from build123d import *

# Parameters (mm, degrees)
SKETCH_1_R          = 27.5
EXTRUDE_1_DEPTH     = 10
EXTRUDE_2_DEPTH     = 16
CUT_EXTRUDE_3_DEPTH = 20
FILLET_3_R          = 2
SKETCH_7_W          = 2
SKETCH_7_H          = 5
SKETCH_7_W_2        = 5
SKETCH_7_H_2        = 2
CUT_EXTRUDE_4_DEPTH = 20
SKETCH_8_R          = 1.75
CUT_EXTRUDE_5_DEPTH = 20
SKETCH_9_R          = 1.75
CUT_EXTRUDE_6_DEPTH = 30.5


with BuildPart() as part:
    # 草图1 → 凸台-拉伸1 (new body)
    with BuildSketch(Plane.XY):
        Circle(SKETCH_1_R)
    extrude(amount=EXTRUDE_1_DEPTH)

    # 草图2 → 凸台-拉伸2 (add)
    with BuildSketch(Plane.XY.offset(10)):
        with BuildLine():
            Line((-2.5, 5.5), (-2.5, 17.5))
            Line((-2.5, 17.5), (-2.5, 18.792973669))
            ThreePointArc((-2.5, 18.792973669), (-13.405705116, 13.405705116), (-18.792973669, 2.5))
            Line((-18.792973669, 2.5), (-17.5, 2.5))
            Line((-17.5, 2.5), (-5.5, 2.5))
            ThreePointArc((-5.5, 2.5), (-3.378679656, 3.378679656), (-2.5, 5.5))
        make_face()
        with BuildLine():
            Line((17.5, -2.5), (5.5, -2.5))
            ThreePointArc((5.5, -2.5), (3.378679656, -3.378679656), (2.5, -5.5))
            Line((2.5, -5.5), (2.5, -17.5))
            Line((2.5, -17.5), (2.5, -18.792973669))
            ThreePointArc((2.5, -18.792973669), (13.405705116, -13.405705116), (18.792973669, -2.5))
            Line((18.792973669, -2.5), (17.5, -2.5))
        make_face()
        with BuildLine():
            Line((17.5, 2.5), (5.5, 2.5))
            ThreePointArc((5.5, 2.5), (3.378679656, 3.378679656), (2.5, 5.5))
            Line((2.5, 5.5), (2.5, 17.5))
            Line((2.5, 17.5), (2.5, 18.792973669))
            ThreePointArc((2.5, 18.792973669), (13.405705116, 13.405705116), (18.792973669, 2.5))
            Line((18.792973669, 2.5), (17.5, 2.5))
        make_face()
        with BuildLine():
            Line((-2.5, -17.5), (-2.5, -5.5))
            ThreePointArc((-2.5, -5.5), (-3.378679656, -3.378679656), (-5.5, -2.5))
            Line((-5.5, -2.5), (-17.5, -2.5))
            Line((-17.5, -2.5), (-18.792973669, -2.5))
            ThreePointArc((-18.792973669, -2.5), (-13.405705116, -13.405705116), (-2.5, -18.792973669))
            Line((-2.5, -18.792973669), (-2.5, -17.5))
        make_face()
    extrude(amount=EXTRUDE_2_DEPTH)

    # 草图6 → 切除-拉伸3 (cut)
    with BuildSketch(Plane.XY.offset(10)):
        Polygon((18.792973669, -2.5), (5.5, -2.5), (2.5, -2.5), (2.5, -5.5), (2.5, -18.792973669), (-2.5, -18.792973669), (-2.5, -5.5), (-2.5, -2.5), (-5.5, -2.5), (-18.792973669, -2.5), (-18.792973669, 2.5), (-5.5, 2.5), (-2.5, 2.5), (-2.5, 5.5), (-2.5, 18.792973669), (2.5, 18.792973669), (2.5, 5.5), (2.5, 2.5), (5.5, 2.5), (18.792973669, 2.5), align=None)
    extrude(amount=-CUT_EXTRUDE_3_DEPTH, mode=Mode.SUBTRACT)

    # 圆角3
    # the kernel refuses this fillet: 2 mm, written as the material it adds along each edge
    with BuildSketch(Plane(origin=(0, 0, 10), x_dir=(-0.13117570134694587, -0.9913591354177037, 0), z_dir=(-0.9913591354177037, 0.13117570134694587, 0))) as fillet_3_piece_1_section:
        with BuildLine():
            CenterArc((18.958529988 + FILLET_3_R, FILLET_3_R), FILLET_3_R, 180, 90)
            Line((18.958529988, FILLET_3_R), (18.958529988, 0))
            Line((18.958529988, 0), (18.958529988 + FILLET_3_R, 0))
        make_face()
    fillet_3_piece_1 = revolve(axis=Axis((0, 0, 10), (0, 0, 1)), revolution_arc=105.075073745, mode=Mode.PRIVATE)
    fillet_3_piece_1 = split(fillet_3_piece_1, bisect_by=Plane(origin=(2.5, -19.248904349, 10.242638579), z_dir=(1, 0, 0)), keep=Keep.TOP, mode=Mode.PRIVATE)
    fillet_3_piece_1 = split(fillet_3_piece_1, bisect_by=Plane(origin=(4.206837789, -2.5, 10.242638579), z_dir=(0, -1, 0)), keep=Keep.TOP, mode=Mode.PRIVATE)
    add(fillet_3_piece_1)
    with BuildSketch(Plane(origin=(0, 0, 10), x_dir=(-0.13117570134694623, 0.9913591354177035, 0), z_dir=(-0.9913591354177035, -0.13117570134694623, 0))) as fillet_3_piece_2_section:
        with BuildLine():
            CenterArc((18.958529988 + FILLET_3_R, -FILLET_3_R), FILLET_3_R, 90, 90)
            Line((18.958529988, -FILLET_3_R), (18.958529988, 0))
            Line((18.958529988, 0), (18.958529988 + FILLET_3_R, 0))
        make_face()
    fillet_3_piece_2 = revolve(axis=Axis((0, 0, 10), (0, 0, -1)), revolution_arc=105.075073745, mode=Mode.PRIVATE)
    fillet_3_piece_2 = split(fillet_3_piece_2, bisect_by=Plane(origin=(4.206838505, 2.5, 10.242637951), z_dir=(0, 1, 0)), keep=Keep.TOP, mode=Mode.PRIVATE)
    fillet_3_piece_2 = split(fillet_3_piece_2, bisect_by=Plane(origin=(2.5, 19.24890412, 10.242637951), z_dir=(1, 0, 0)), keep=Keep.TOP, mode=Mode.PRIVATE)
    add(fillet_3_piece_2)
    with BuildSketch(Plane(origin=(0, 0, 10), x_dir=(-0.9913591354177035, 0.13117570134694678, 0), z_dir=(0.13117570134694678, 0.9913591354177035, 0))) as fillet_3_piece_3_section:
        with BuildLine():
            CenterArc((18.958529988 + FILLET_3_R, FILLET_3_R), FILLET_3_R, 180, 90)
            Line((18.958529988, FILLET_3_R), (18.958529988, 0))
            Line((18.958529988, 0), (18.958529988 + FILLET_3_R, 0))
        make_face()
    fillet_3_piece_3 = revolve(axis=Axis((0, 0, 10), (0, 0, 1)), revolution_arc=105.075073745, mode=Mode.PRIVATE)
    fillet_3_piece_3 = split(fillet_3_piece_3, bisect_by=Plane(origin=(-19.248904349, -2.5, 10.242638579), z_dir=(0, -1, 0)), keep=Keep.TOP, mode=Mode.PRIVATE)
    fillet_3_piece_3 = split(fillet_3_piece_3, bisect_by=Plane(origin=(-2.5, -4.206837789, 10.242638579), z_dir=(-1, 0, 0)), keep=Keep.TOP, mode=Mode.PRIVATE)
    add(fillet_3_piece_3)
    with BuildSketch(Plane(origin=(0, 0, 10), x_dir=(0.13117570134694595, 0.9913591354177037, 0), z_dir=(0.9913591354177037, -0.13117570134694595, 0))) as fillet_3_piece_4_section:
        with BuildLine():
            CenterArc((18.958529988 + FILLET_3_R, FILLET_3_R), FILLET_3_R, 180, 90)
            Line((18.958529988, FILLET_3_R), (18.958529988, 0))
            Line((18.958529988, 0), (18.958529988 + FILLET_3_R, 0))
        make_face()
    fillet_3_piece_4 = revolve(axis=Axis((0, 0, 10), (0, 0, 1)), revolution_arc=105.075073745, mode=Mode.PRIVATE)
    fillet_3_piece_4 = split(fillet_3_piece_4, bisect_by=Plane(origin=(-2.5, 19.248904349, 10.242638579), z_dir=(-1, 0, 0)), keep=Keep.TOP, mode=Mode.PRIVATE)
    fillet_3_piece_4 = split(fillet_3_piece_4, bisect_by=Plane(origin=(-4.206837789, 2.5, 10.242638579), z_dir=(0, 1, 0)), keep=Keep.TOP, mode=Mode.PRIVATE)
    add(fillet_3_piece_4)

    # 草图7 → 切除-拉伸4 (cut)
    with BuildSketch(Plane(origin=(0, 0, 0), x_dir=(-1, 0, 0), z_dir=(0, 0, -1))):
        with Locations((19.792973669, 0)):
            Rectangle(SKETCH_7_W, SKETCH_7_H)
        with Locations((0, -19.792973669)):
            Rectangle(SKETCH_7_W_2, SKETCH_7_H_2)
        with Locations((-19.792973669, 0)):
            Rectangle(SKETCH_7_W, SKETCH_7_H)
        with Locations((0, 19.792973669)):
            Rectangle(SKETCH_7_W_2, SKETCH_7_H_2)
    extrude(amount=-CUT_EXTRUDE_4_DEPTH, mode=Mode.SUBTRACT)

    # 草图8 → 切除-拉伸5 (cut)
    with BuildSketch(Plane.XY.offset(10)):
        with Locations((0, 24.460175936)):
            Circle(SKETCH_8_R)
        with Locations((24.460175936, 0)):
            Circle(SKETCH_8_R)
        with Locations((0, -24.460175936)):
            Circle(SKETCH_8_R)
        with Locations((-24.460175936, 0)):
            Circle(SKETCH_8_R)
    extrude(amount=-CUT_EXTRUDE_5_DEPTH, mode=Mode.SUBTRACT)

    # 草图9 → 切除-拉伸6 (cut, symmetric)
    with BuildSketch(Plane(origin=(0, 0, 0), x_dir=(1, 0, 0), z_dir=(0, 1, 0))):
        with Locations(Location((-10.646486834, -19, 0), (0, 0, 270))):
            Circle(SKETCH_9_R)
        with Locations(Location((10.646486834, -19, 0), (0, 0, 270))):
            Circle(SKETCH_9_R)
    extrude(amount=CUT_EXTRUDE_6_DEPTH, both=True, mode=Mode.SUBTRACT)


solid = part.part
Can you work these out from the model? Positions are in its coordinate system, mm. A direction names the side the tool comes from. Round coordinates to 2 decimals unless told otherwise and drop trailing zeros. Order: outer loops, then holes, each group sorted by start corner. A loop starts at its lowest first (then second) coordinate and runs counter-clockwise, first axis right, second up. Notation, with made-up numbers: M -1,-7 L 44,-7 A18 cw 44,13 Z; hole C -15.75,44.25 d2. An arc over 180 degrees is marked long. Use a Markdown table: item, result.
1) On a 3-axis mill with a long thin cutter (end or side, diameter ignored), from which of +Z, -Z, +X, -X, +Y, -Y can I reach the whole of each face in a straight line? I mean faces 4 (the face through (-9, -9, 26)), 5 (the face through (13.28, 13.53, 18.9)), 6 (the face through (3, 3, 10)), 7 (the face through (-12, 2.5, 10)), 8 (the face through (-8.91, -9.52, 18.77)). Say none if no direction works.
Geometry says:
| item | result |
|---|---|
| face 4 | +Z, +X, -X, +Y, -Y |
| face 5 | +Z, +X, +Y |
| face 6 | +Z |
| face 7 | +Z, -Z |
| face 8 | +Y, -Y |
2) I'm going to push flat-ended pins straight in: P1, Ø2, axis at x = 10.65, z = 19, coming from the +Y side; P2, Ø12, axis at x = 8.5, z = 10, coming from the +Y side; P3, Ø6, axis at y = -18.5, z = 21, coming from the +X side; P4, Ø1.5, axis at y = 22, z = 4.5, coming from the -X side. Where does each tip first touch, or does it pass through?
Geometry says:
| item | result |
|---|---|
| P1 | passes through |
| P2 | stops at y = 27.39 |
| P3 | stops at x = 10.92 |
| P4 | stops at x = -17.46 |
3) If I drill on line 1 along Y through (x, z) = (0, 5.5); line 2 along X through (y, z) = (10.25, 19); line 3 along Y through (x, z) = (-0.5, 3.75), over which ranges is the centre line in solid material (lowest first)?
Geometry says:
| item | result |
|---|---|
| line 1 | y = -27.5 to -26.21, -22.71 to -20.79, 20.79 to 22.71, 26.21 to 27.5 |
| line 2 | x = -15.95 to -12.4, -8.9 to -2.5, 2.5 to 8.9, 12.4 to 15.95 |
| line 3 | y = -27.5 to -26.14, -22.78 to -20.79, 20.79 to 22.78, 26.14 to 27.5 |
4) Imagine slicing it at C-C (z = 19). Give the number of separate pieces and of enclosed holes in the cut face, then the cut area to 3 significant figures.
Geometry says:
| item | result |
|---|---|
| separate pieces | 8 |
| enclosed holes | 0 |
| area | 584 mm² |
5) If we mould it in two halves opening along Y, with no side actions, what happens to faces 1 (the face through (-13.28, 13.53, 18.9)), 2 (the face through (-13.53, -13.28, 18.9)), 3 (the face through (0, -20.793, 5))? For each: +Y half, -Y half, draft (parallel to the pull), parting line (faces both ways), or undercut.
Geometry says:
| item | result |
|---|---|
| face 1 | +Y half |
| face 2 | -Y half |
| face 3 | undercut |
6) Imagine slicing it at D-D (z = 4). List the corners of the cut face in (x, y) for me, then the cut area to 3 significant figures.
Geometry says:
| item | result |
|---|---|
| outline | C 0,0 d55; hole C -24.46,0 d3.5; hole M -20.79,-2.5 L -2.5,-2.5 L -2.5,-20.79 L 2.5,-20.79 L 2.5,-2.5 L 20.79,-2.5 L 20.79,2.5 L 2.5,2.5 L 2.5,20.79 L -2.5,20.79 L -2.5,2.5 L -20.79,2.5 Z; hole C 0,-24.46 d3.5; hole C 0,24.46 d3.5; hole C 24.46,0 d3.5 |
| area | 1,950 mm² |
7) Imagine slicing it at A-A (y = 0). List the corners of the cut face in (x, z) for me.
Geometry says:
| item | result |
|---|---|
| outline | M -27.5,0 L -26.21,0 L -26.21,10 L -27.5,10 Z; M -22.71,0 L -20.79,0 L -20.79,10 L -22.71,10 Z; M 20.79,0 L 22.71,0 L 22.71,10 L 20.79,10 Z; M 26.21,0 L 27.5,0 L 27.5,10 L 26.21,10 Z |
